Could you check a few things on this model? Use its own coordinates, in mm. Face numbers are marked on the shaded views. A direction names the side the tool comes from. Give positions to 0.01 mm unless a question says otherwise; leave off trailing zeros. Loops run counter-clockwise (first coordinate to the right, second up) from the corner with the lowest first, then second, coordinate; pieces in that order, holes last. Notation, with made-up numbers: M 4.25,12.25 L 9.25,12.25 A27 ccw 9.25,43.25 Z; hole C 18.5,-17 d9. An arc over 180 degrees is marked long. Return JSON: item names as keys, results as strings. Group by question number.
1. If we section it at C-C (z = 9): Write out the boundary of the cut face in (x, y).
2. For the marked faces 1 and 2, which set-ups out of +Z, -Z, +X, -X, +Y, -Y let a thin tool reach every point of the face, with its end or its side?
3. If we section it at D-D (x = -6.75): Write out the boundary of the cut face in (y, z).
4. For pin 1 (1.5 mm diameter, centred on x = -17, y = -10.5, fed in from -Z); pin 2 (5 mm diameter, centred on y = 0, z = 9, fed in from +X), each with a flat end and sliding along its axis, tell me the tip position at first contact or that it passes through.
5. If we section it at B-B (x = -12.5): Write out the boundary of the cut face in (y, z).
6. Please list where these lines run through material, in increasing order: line 1 (Y direction, x = -4.25, z = 9); line 2 (Y direction, x = -9, z = 9); line 3 (X direction, y = -12.5, z = 5.25).
7. If we section it at A-A (y = 0): Write out the boundary of the cut face in (x, z).
8. If we mould it in two halves opening along Y, with no side actions, what happens to the marked faces 3, 4, 5 and 6? For each: +Y half, -Y half, draft (parallel to the pull), parting line (faces both ways), or undercut.
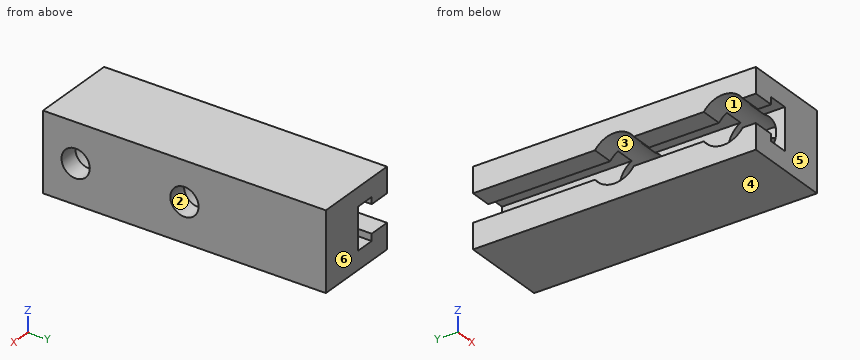
Autodesk Inventor part; units mm, degrees
ref_plane "YZ Plane" through (0, 0, 0) normal (1, 0, 0) x (0, 1, 0)
ref_plane "XZ Plane" through (0, 0, 0) normal (0, 1, 0) x (-1, 0, 0)
ref_plane "XY Plane" through (0, 0, 0) normal (0, 0, 1) x (1, 0, 0)
sketch "Sketch1" plane through (0, 0, 0) normal (0, 1, 0) x (-1, 0, 0)
  line L0 (0, 0) -> (20, 0)
  line L1 (20, 0) -> (20, 18)
  line L2 (20, 18) -> (0, 18)
  line L3 (0, 18) -> (0, 0)
  dimension "d0" = 18
  dimension "d1" = 20
extrude "Extrusion1" add sketch "Sketch1" along normal mid plane 65
sketch "Sketch2" plane through (-20, -32.5, 18) normal (-1, 0, 0) x (0, 0, 1)
  circle A0 centre (-9, 7.5) radius 3.25
  circle A1 centre (-9, 32.5) radius 3.25
  circle A2 centre (-9, 7.5) radius 5.5
  circle A3 centre (-9, 32.5) radius 5.5
  line L0 (0, 0) -> (-18, 0)
  line L1 (-18, 32.5) -> (8.866, 32.5) construction
  line L2 (-9, 65.0931) -> (-9, 0) construction
  dimension "d4" = 6.5
  dimension "d5" = 6.5
  dimension "d8" = 11
  dimension "d9" = 11
  dimension "d34" = 25
extrude "Extrusion2" cut sketch "Sketch2" against normal through all contours A0 | A1
extrude "Extrusion3" cut sketch "Sketch2" against normal blind 15.5
sketch "Sketch4" plane through (0, 32.5, 0) normal (0, 1, 0) x (1, 0, 0)
  line L0 (-20, 0) -> (-20, -18)
  line L1 (-20, -9) -> (2.4786, -9) construction
  line L2 (-20, -12.2) -> (-15, -12.2)
  line L3 (-15, -12.2) -> (-15, -13.8)
  line L4 (-15, -13.8) -> (-10.5, -13.8)
  line L5 (-10.5, -13.8) -> (-10.5, -4.2)
  line L6 (-10.5, -4.2) -> (-15, -4.2)
  line L7 (-15, -4.2) -> (-15, -5.8)
  line L8 (-15, -5.8) -> (-20, -5.8)
  line L9 (-20, -12.2) -> (-20, -5.8)
  point P0 (0, 0)
  dimension "d28" = 6.4
  dimension "d29" = 4.5
  dimension "d30" = 9.6
  dimension "d31" = 5
extrude "Extrusion4" cut sketch "Sketch4" against normal through all
properties part number "HeadbarHolderBracketAdjustable20mm" material "Aluminum 6061"
Answer:
{
 "1": {"outline": "M -10.5,-32.5 L 0,-32.5 L 0,-28.25 L -4.5,-28.25 L -4.5,-30.5 L -10.5,-30.5 Z; M -10.5,-19.5 L -4.5,-19.5 L -4.5,-21.75 L 0,-21.75 L 0,-3.25 L -4.5,-3.25 L -4.5,-5.5 L -10.5,-5.5 Z; M -10.5,5.5 L -4.5,5.5 L -4.5,3.25 L 0,3.25 L 0,32.5 L -10.5,32.5 Z"},
 "2": {"face 1": "-X", "face 2": "+X, -X"},
 "3": {"outline": "M -32.5,0 L 32.5,0 L 32.5,18 L -32.5,18 Z; hole C -25,9 d11; hole C 0,9 d11"},
 "4": {"pin 1": "stops at z = 0", "pin 2": "passes through"},
 "5": {"outline": "M -32.5,0 L 32.5,0 L 32.5,4.2 L 2.69,4.2 A5.5 cw -2.69,4.2 L -22.31,4.2 A5.5 cw -27.69,4.2 L -32.5,4.2 Z; M -32.5,13.8 L -27.69,13.8 A5.5 cw -22.31,13.8 L -2.69,13.8 A5.5 cw 2.69,13.8 L 32.5,13.8 L 32.5,18 L -32.5,18 Z"},
 "6": {"line 1": "y = -32.5 to -28.25, -21.75 to -3.25, 3.25 to 32.5", "line 2": "y = -32.5 to -30.5, -19.5 to -5.5, 5.5 to 32.5", "line 3": "x = -20 to -15, -10.5 to 0"},
 "7": {"outline": "M -20,0 L 0,0 L 0,5.75 L -4.5,5.75 L -4.5,3.5 L -20,3.5 Z; M -20,14.5 L -4.5,14.5 L -4.5,12.25 L 0,12.25 L 0,18 L -20,18 Z"},
 "8": {"face 3": "undercut", "face 4": "draft", "face 5": "-Y half", "face 6": "+Y half"}
}
